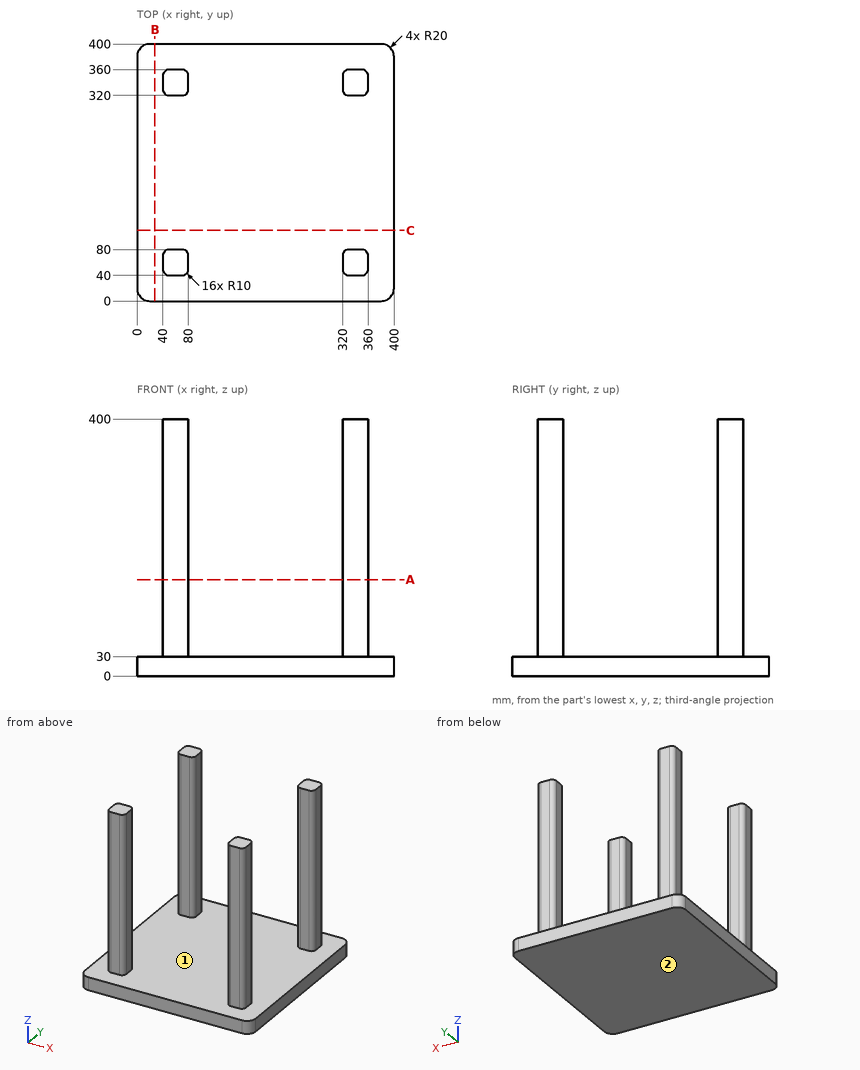
Part print with two shaded views. Sizes in mm from the minimum x, y, z corner. A direction names the side the tool comes from. Round coordinates to 2 decimals unless told otherwise and drop trailing zeros. Order: outer loops, then holes, each group sorted by start corner. A loop starts at its lowest first (then second) coordinate and runs counter-clockwise, first axis right, second up. Notation, with made-up numbers: (88.5, -32.5) - (126.5, -32.5) arc R20 cw to (126.5, -20.5) - close; hole circle Ø5 at (69, 17.5). An arc over 180 degrees is marked (long way). Answer as CSV lines item,"result". Start each with the question number.
1. Tool access for the marked faces 1 and 2: list every direction of +Z, -Z, +X, -X, +Y, -Y with a clear straight run to the whole face (end or side of a thin tool).
2. Saw through at A-A, the plane z = 150. Count the separate pieces of the cut face and the enclosed holes in it, and give its area (3 significant figures).
3. Drill centre lines: L1, parallel to Y at x = 341.5, z = 165; L2, parallel to Z at x = 238, y = 83; L3, parallel to X at y = 325, z = 186. Where is each one in solid material? Low to high. Write a range as [from, to].
4. Pin check, flat tips, straight feed: pin 1 (22 mm diameter, centred on y = 337.5, z = 257.5, fed in from +X); pin 2 (22 mm diameter, centred on x = 63.5, z = 150, fed in from -Y); pin 3 (10 mm diameter, centred on y = 335.5, z = 244.5, fed in from -X); pin 4 (1 mm diameter, centred on x = 253.5, y = 208, fed in from -Z). Stop position of each tip, or through.
5. Saw through at B-B, the plane x = 28. Write the cut outline in (y, z), and give its area (3 significant figures).
Model answer:
1,face 1,"+Z"
1,face 2,"-Z, +X, -X, +Y, -Y"
2,separate pieces,"4"
2,enclosed holes,"0"
2,area,"6,060 mm²"
3,L1,"y = [40, 80], [320, 360]"
3,L2,"z = [0, 30]"
3,L3,"x = [41.34, 78.66], [321.34, 358.66]"
4,pin 1,"stops at x = 360"
4,pin 2,"stops at y = 40"
4,pin 3,"stops at x = 40"
4,pin 4,"stops at z = 0"
5,outline,"(0, 0) - (400, 0) - (400, 30) - (0, 30) - close"
5,area,"12,000 mm²"
